CAD build for the part. Positions are in the model's coordinates, mm. Give positions to 0.01 mm unless a question says otherwise; leave off trailing zeros. Loops run counter-clockwise (first coordinate to the right, second up) from the corner with the lowest first, then second, coordinate; pieces in that order, holes last. Notation, with made-up numbers: M 63,-18.5 L 74,-18.5 A16 ccw 74,-11.5 Z; hole C 20.5,48.5 d11. An arc over 180 degrees is marked long. One line per question, with ' | ' between items.
```python
from build123d import *

# Parameters (mm, degrees)
SKETCH1_W               = 170
SKETCH1_H               = 40
BOSS_EXTRUDE1_DEPTH     = 1.5
SKETCH2_R               = 1.5
CUT_EXTRUDE1_DEPTH      = 15
CUT_EXTRUDE1_DEPTH_BACK = 15


with BuildPart() as part:
    # Sketch1 → Boss-Extrude1 (new body)
    with BuildSketch(Plane(origin=(0, 0, 0), x_dir=(0, 0, -1), z_dir=(1, 0, 0))):
        with Locations((85, 20)):
            Rectangle(SKETCH1_W, SKETCH1_H)
    extrude(amount=BOSS_EXTRUDE1_DEPTH)

    # Sketch2 → Cut-Extrude1 (cut, two sides)
    with BuildSketch(Plane(origin=(1.5, 0, 0), x_dir=(0, 0, -1), z_dir=(1, 0, 0))) as cut_extrude1_sk:
        with Locations((18, 6.5)):
            Circle(SKETCH2_R)
        with Locations((152, 6.5)):
            Circle(SKETCH2_R)
        with Locations((163.5, 33.5)):
            Circle(SKETCH2_R)
        with Locations((6.5, 33.5)):
            Circle(SKETCH2_R)
    extrude(amount=CUT_EXTRUDE1_DEPTH, mode=Mode.SUBTRACT)
    extrude(cut_extrude1_sk.sketch, amount=-CUT_EXTRUDE1_DEPTH_BACK, mode=Mode.SUBTRACT)


solid = part.part
```
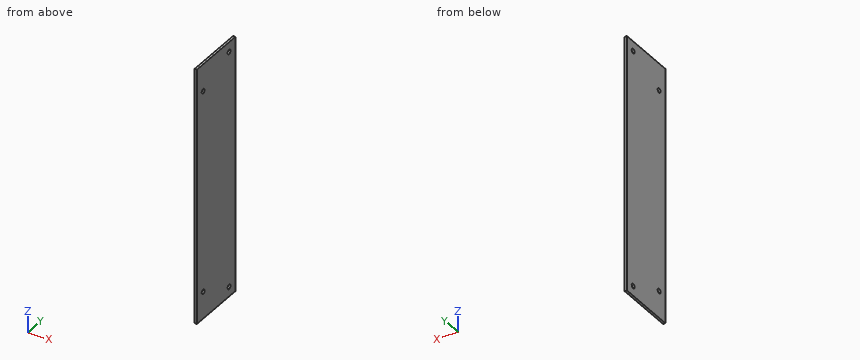
Item 1: Saw through at A-A on z = -6.5. Give the cut face in (x, y).
Conclusion:
outline: M 0,0 L 1.5,0 L 1.5,32 L 0,32 Z; M 0,35 L 1.5,35 L 1.5,40 L 0,40 Z
Item 2: Saw through at B-B on y = 33.5. Give the cut face in (x, z), and give its area (3 significant figures).
Conclusion:
outline: M 0,-170 L 1.5,-170 L 1.5,-165 L 0,-165 Z; M 0,-162 L 1.5,-162 L 1.5,-8 L 0,-8 Z; M 0,-5 L 1.5,-5 L 1.5,0 L 0,0 Z | area: 246 mm²
Item 3: Drill centre lines: line 1 along Y through (x, z) = (1.05, -18); line 2 along Y through (x, z) = (1.1, -163.5); line 3 along Z through (x, y) = (1.4, 34.5). Where is each one in solid material? Low to high. Write a range as [from, to].
Conclusion:
line 1: [0, 5], [8, 40] | line 2: [0, 32], [35, 40] | line 3: [-170, -164.62], [-162.38, -7.62], [-5.38, 0]
